Verification items for the finished model (mm, model axes). A direction names the side the tool comes from. Give positions to 0.01 mm unless a question says otherwise; leave off trailing zeros. Write each loop counter-clockwise with the first axis right and the second up, starting at its lowest first coordinate (ties: lowest second). Pieces come first, ordered by that corner, then holes. Notation, with made-up numbers: (51.25, 35.25) -> (75.25, 35.25) arc R16 ccw to (75.25, 64.25) -> close; hole circle Ø6 at (-21, 6.5). An arc over 180 degrees is marked (long way). Write item = value, one per line.
from build123d import *

# Parameters (mm, degrees)
SKETCH_W        = 290
SKETCH_H        = 130
PAD_DEPTH       = 2.5
SKETCH001_R     = 2.5
POCKET_DEPTH    = 5.001
SKETCH002_W     = 5
SKETCH002_H     = 10
POCKET001_DEPTH = 5.001
SKETCH003_W     = 10
SKETCH003_H     = 5
PAD001_DEPTH    = 5
SKETCH004_W     = 10
SKETCH004_H     = 5
POCKET002_DEPTH = 5.001
SKETCH005_W     = 5
SKETCH005_H     = 10
POCKET003_DEPTH = 5.001
SKETCH006_R     = 2.5
POCKET004_DEPTH = 5.001


with BuildPart() as part:
    # Sketch → Pad (new body, symmetric)
    with BuildSketch(Plane.XY):
        with Locations((145, 65)):
            Rectangle(SKETCH_W, SKETCH_H)
    extrude(amount=PAD_DEPTH, both=True)

    # Sketch001 (on Face6 of Pad) → Pocket (cut, through all)
    with BuildSketch(Plane.XY.offset(2.5)):
        with Locations((15, 110)):
            Circle(SKETCH001_R)
        with Locations((15, 15)):
            Circle(SKETCH001_R)
    extrude(amount=-POCKET_DEPTH, mode=Mode.SUBTRACT)

    # Sketch002 (on Face5 of Pocket) → Pocket001 (cut, through all)
    with BuildSketch(Plane.XY.offset(2.5)):
        with Locations((287.5, 15)):
            Rectangle(SKETCH002_W, SKETCH002_H)
        with Locations((287.5, 35)):
            Rectangle(SKETCH002_W, SKETCH002_H)
        with Locations((287.5, 55)):
            Rectangle(SKETCH002_W, SKETCH002_H)
        with Locations((287.5, 75)):
            Rectangle(SKETCH002_W, SKETCH002_H)
        with Locations((287.5, 95)):
            Rectangle(SKETCH002_W, SKETCH002_H)
        with Locations((287.5, 115)):
            Rectangle(SKETCH002_W, SKETCH002_H)
    extrude(amount=-POCKET001_DEPTH, mode=Mode.SUBTRACT)

    # Sketch003 (on Face5 of Pocket001) → Pad001 (join)
    with BuildSketch(Plane.XY.offset(2.5)):
        with Locations((5, 132.5)):
            Rectangle(SKETCH003_W, SKETCH003_H)
        with Locations((25, 132.5)):
            Rectangle(SKETCH003_W, SKETCH003_H)
        with Locations((45, 132.5)):
            Rectangle(SKETCH003_W, SKETCH003_H)
        with Locations((65, 132.5)):
            Rectangle(SKETCH003_W, SKETCH003_H)
        with Locations((85, 132.5)):
            Rectangle(SKETCH003_W, SKETCH003_H)
        with Locations((105, 132.5)):
            Rectangle(SKETCH003_W, SKETCH003_H)
        with Locations((125, 132.5)):
            Rectangle(SKETCH003_W, SKETCH003_H)
        with Locations((145, 132.5)):
            Rectangle(SKETCH003_W, SKETCH003_H)
        with Locations((165, 132.5)):
            Rectangle(SKETCH003_W, SKETCH003_H)
        with Locations((185, 132.5)):
            Rectangle(SKETCH003_W, SKETCH003_H)
        with Locations((205, 132.5)):
            Rectangle(SKETCH003_W, SKETCH003_H)
        with Locations((225, 132.5)):
            Rectangle(SKETCH003_W, SKETCH003_H)
        with Locations((245, 132.5)):
            Rectangle(SKETCH003_W, SKETCH003_H)
        with Locations((265, 132.5)):
            Rectangle(SKETCH003_W, SKETCH003_H)
    extrude(amount=-PAD001_DEPTH)

    # Sketch004 (on Face86 of Pad001) → Pocket002 (cut, through all)
    with BuildSketch(Plane.XY.offset(2.5)):
        with Locations((15, 2.5)):
            Rectangle(SKETCH004_W, SKETCH004_H)
        with Locations((35, 2.5)):
            Rectangle(SKETCH004_W, SKETCH004_H)
        with Locations((55, 2.5)):
            Rectangle(SKETCH004_W, SKETCH004_H)
        with Locations((75, 2.5)):
            Rectangle(SKETCH004_W, SKETCH004_H)
        with Locations((95, 2.5)):
            Rectangle(SKETCH004_W, SKETCH004_H)
        with Locations((115, 2.5)):
            Rectangle(SKETCH004_W, SKETCH004_H)
    extrude(amount=-POCKET002_DEPTH, mode=Mode.SUBTRACT)

    # Sketch005 (on Face4 of Pocket002) → Pocket003 (cut, through all)
    with BuildSketch(Plane.XY.offset(2.5)):
        with Locations((127.5, 15)):
            Rectangle(SKETCH005_W, SKETCH005_H)
        with Locations((127.5, 35)):
            Rectangle(SKETCH005_W, SKETCH005_H)
        with Locations((127.5, 55)):
            Rectangle(SKETCH005_W, SKETCH005_H)
        with Locations((127.5, 75)):
            Rectangle(SKETCH005_W, SKETCH005_H)
        with Locations((127.5, 95)):
            Rectangle(SKETCH005_W, SKETCH005_H)
        with Locations((127.5, 115)):
            Rectangle(SKETCH005_W, SKETCH005_H)
    extrude(amount=-POCKET003_DEPTH, mode=Mode.SUBTRACT)

    # Sketch006 (on Face4 of Pocket003) → Pocket004 (cut, through all)
    with BuildSketch(Plane.XY.offset(2.5)):
        with Locations((20, 67.5)):
            Circle(SKETCH006_R)
        with Locations((109.8, 67.5)):
            Circle(SKETCH006_R)
    extrude(amount=-POCKET004_DEPTH, mode=Mode.SUBTRACT)


solid = part.part
Item 1: Set-up check for faces 4 (the flat face through (287, 90, 0)), 5 (the flat face through (110, 2, 0)), 6 (the flat face through (160, 132, 0)): record each of +Z, -Z, +X, -X, +Y, -Y from which the full face is reachable in a straight line by a thin tool's end or side.
Response values:
face_4 = +Z, -Z, +X
face_5 = +Z, -Z, -Y
face_6 = +Z, -Z, +Y
Item 2: Sectioned sample at B-B on z = -1.65. Give the number of separate pieces and of enclosed holes in the cut face, then the cut area to 3 significant figures.
Response values:
separate_pieces = 1
enclosed_holes = 10
area = 37,400 mm^2
Item 3: Material ranges on line 1 (Y direction, x = 15, z = -1.05); line 2 (X direction, y = 96, z = -1.65); line 3 (Y direction, x = 178.5, z = -1.8), recorded low to high.
Response values:
line_1 = 5 to 12.5, 17.5 to 107.5, 112.5 to 130
line_2 = 0 to 125, 130 to 285
line_3 = 0 to 130
Item 4: Sectioned sample at C-C on x = 136. Record the cut outline in (y, z).
Response values:
outline = (0, -2.5) -> (130, -2.5) -> (130, 2.5) -> (0, 2.5) -> close
Item 5: Sectioned sample at A-A on y = 53. Record the cut outline in (x, z), then the cut area to 3 significant figures.
Response values:
outline = (0, -2.5) -> (125, -2.5) -> (125, 2.5) -> (0, 2.5) -> close; (130, -2.5) -> (285, -2.5) -> (285, 2.5) -> (130, 2.5) -> close
area = 1,400 mm^2
Item 6: Go/stop test with flat-tipped pins: P1, Ø2.5, axis at y = 131.5, z = 1, coming from the -X side; P2, Ø2.5, axis at y = 133.5, z = 0, coming from the +X side; P3, Ø2.5, axis at x = 14.5, z = -1, coming from the +Y side; P4, Ø2.5, axis at y = 77.5, z = 0.5, coming from the +X side. Record where each tip stops, or that it passes through.
Response values:
P1 = 0
P2 = 270
P3 = 130
P4 = 285
Item 7: Mould release check, pull along Y, two halves, no side actions. Record for faces 1 (the flat face through (290, 25, 0)), 2 (the flat face through (127, 110, 0)), 3 (the flat face through (155, 130, 0)): +Y half, -Y half, draft (parallel to the pull), parting line (faces both ways), or undercut.
Response values:
face_1 = draft
face_2 = undercut
face_3 = +Y half
